Verification items for this drawing (mm, ordinates from the low corner). Round coordinates to 2 decimals unless told otherwise and drop trailing zeros. Loops run counter-clockwise (first coordinate to the right, second up) from the corner with the lowest first, then second, coordinate; pieces in that order, holes last. Notation, with made-up numbers: (52, -32) - (101, -32) arc R13 cw to (101, -24) - close; hole circle Ø5 at (82.5, -33). An arc over 180 degrees is marked (long way). Put each result on its own line as item: value. Start each with the question number.
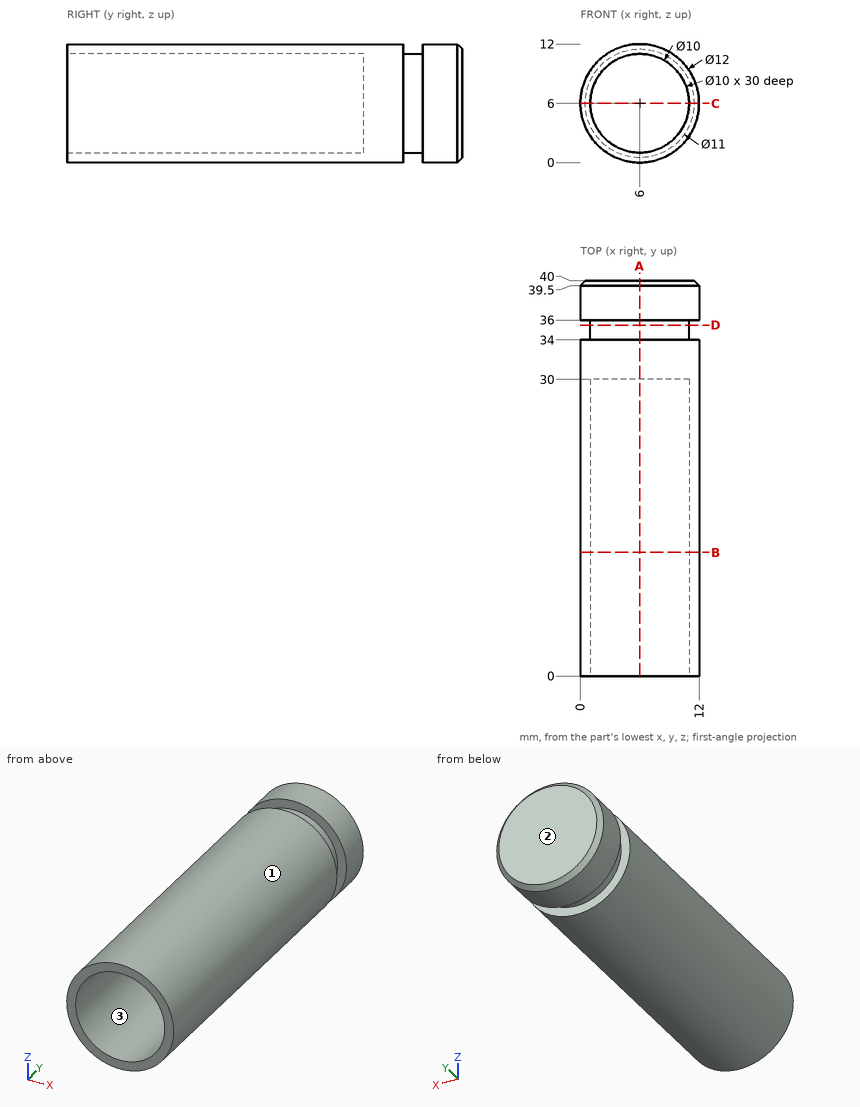
Q1. Cross-section at C-C on z = 6. Enter the section's corners in (x, y), and give its area (3 significant figures).
Q2. Material ranges on line 1 (X direction, y = 19.25, z = 6); line 2 (Y direction, x = 7, z = 2); line 3 (Y direction, x = 1, z = 5), recorded low to high. Write a range as from..to.
Q3. Depth check by flat-ended pin: pin 1 Ø1.5 at (x, z) = (8, 8.5) entering from -Y; pin 2 Ø4 at (y, z) = (11.5, 3.5) entering from +X; pin 3 Ø2 at (y, z) = (30, 10.5) entering from +X. Enter the tip coordinate at first touch or a pass-through.
Q4. Cross-section at A-A on x = 6. Enter the section's corners in (y, z).
Q5. Cross-section at B-B on y = 12.5. Enter the section's corners in (x, z), and give its area (3 significant figures).
Q6. Cross-section at D-D on y = 35.5. Enter the section's corners in (x, z).
Q7. Draft check along Z on the marked faces 1, 2 and 3. Enter one of: +Z half, -Z half, draft (parallel to the pull), parting line (faces both ways), or undercut.
Answer list:
1. outline: (0, 0) - (1, 0) - (1, 30) - (11, 30) - (11, 0) - (12, 0) - (12, 34) - (11, 34) - (11, 36) - (12, 36) - (12, 39.5) - (11.5, 40) - (0.5, 40) - (0, 39.5) - (0, 36) - (1, 36) - (1, 34) - (0, 34) - close
1. area: 176 mm2
2. line 1: x = 0..1, 11..12
2. line 2: y = 30..40
2. line 3: y = 0..34, 36..40
3. pin 1: stops at y = 30
3. pin 2: stops at x = 11.98
3. pin 3: stops at x = 10.87
4. outline: (0, 0) - (34, 0) - (34, 1) - (36, 1) - (36, 0) - (39.5, 0) - (40, 0.5) - (40, 11.5) - (39.5, 12) - (36, 12) - (36, 11) - (34, 11) - (34, 12) - (0, 12) - (0, 11) - (30, 11) - (30, 1) - (0, 1) - close
5. outline: circle Ø12 at (6, 6); hole circle Ø10 at (6, 6)
5. area: 34.6 mm2
6. outline: circle Ø10 at (6, 6)
7. face 1: parting line
7. face 2: draft
7. face 3: undercut
